Verification items for the finished model (mm, model axes). A direction names the side the tool comes from. Coordinates: 2 decimals unless noted, no trailing zeros. Write each loop counter-clockwise with the first axis right and the second up, starting at its lowest first coordinate (ties: lowest second). Pieces come first, ordered by that corner, then holes. Notation, with made-up numbers: (-5.5, 2.25) -> (8.5, 2.25) arc R18 cw to (8.5, 6.25) -> close; hole circle Ø6 at (16, 32). An arc over 180 degrees is marked (long way). Answer in a Markdown table with one row per item.
Autodesk Inventor part; units mm, degrees
ref_plane "YZ Plane" through (0, 0, 0) normal (1, 0, 0) x (0, 1, 0)
ref_plane "XZ Plane" through (0, 0, 0) normal (0, 1, 0) x (-1, 0, 0)
ref_plane "XY Plane" through (0, 0, 0) normal (0, 0, 1) x (1, 0, 0)
sketch "스케치1" plane through (0, 0, 0) normal (0, 1, 0) x (-1, 0, 0)
  line L0 (0, 0) -> (11.5, 0)
  line L1 (11.5, 0) -> (11.5, -16.1)
  line L2 (11.5, -16.1) -> (0, -16.1)
  line L3 (0, -16.1) -> (0, 0)
  dimension "d0" = 11.5
  dimension "d1" = 16.1
extrude "돌출1" add sketch "스케치1" along normal blind 0.8
fillet "모깎기1" radius 1 2 edges at (0, 0.4, 0) (-11.5, 0.4, 0)
sketch "스케치2" plane through (0, 0.8, 0) normal (0, 1, 0) x (1, 0, 0)
  line L0 (0, 1) -> (0, 16.1)
  line L1 (0, 16.1) -> (-11.5, 16.1)
  line L2 (-1.5, 16.1) -> (-10, 16.1)
  line L3 (-10, 16.1) -> (-10, 14.6)
  line L4 (-10, 14.6) -> (-1.5, 14.6)
  line L5 (-1.5, 14.6) -> (-1.5, 16.1)
  point P0 (0, 0)
  dimension "d5" = 8.5
  dimension "d6" = 1.5
  dimension "d7" = 1.5
extrude "돌출2" add sketch "스케치2" along normal blind 1
properties part number "Case_Top"
1. Sectioned sample at C-C, the plane y = 1.5. Record the cut outline in (x, z), and give its area (4 significant figures).
Findings below:
| item | result |
|---|---|
| outline | (-10, -16.1) -> (-1.5, -16.1) -> (-1.5, -14.6) -> (-10, -14.6) -> close |
| area | 12.75 mm² |
2. Go/stop test with flat-tipped pins: pin 1 (0.5 mm diameter, centred on x = -4.5, y = 1.5, fed in from +Z); pin 2 (0.5 mm diameter, centred on y = 1, z = -15.5, fed in from +X); pin 3 (0.8 mm diameter, centred on y = 1.5, z = -15.5, fed in from -X). Record where each tip stops, or that it passes through.
Findings below:
| item | result |
|---|---|
| pin 1 | stops at z = -14.6 |
| pin 2 | stops at x = 0 |
| pin 3 | stops at x = -10 |
3. Access from +Z, -Z, +X, -X, +Y, -Y to the whole of each face (thin tool, end or side, straight path). Record for faces 1 (the face through (-1.5, 1, -15)), 2 (the face through (-6, 1, -14.6)), 3 (the face through (-10, 1, -15)), 4 (the face through (-6, 1, -16.1)).
Findings below:
| item | result |
|---|---|
| face 1 | +Z, -Z, +X, +Y |
| face 2 | +Z, +X, -X, +Y |
| face 3 | +Z, -Z, -X, +Y |
| face 4 | -Z, +X, -X, +Y, -Y |
4. Sectioned sample at A-A, the plane x = -5.5. Record the cut outline in (y, z).
Findings below:
| item | result |
|---|---|
| outline | (0, -16.1) -> (1.8, -16.1) -> (1.8, -14.6) -> (0.8, -14.6) -> (0.8, 0) -> (0, 0) -> close |
5. Material ranges on probe 1 along Y at (x, z) = (-2.75, -10.25); probe 2 along X at (y, z) = (1, -14.75); probe 3 along Z at (x, y) = (-5.5, 1.5), recorded low to high. Write a range as from..to.
Findings below:
| item | result |
|---|---|
| probe 1 | y = 0..0.8 |
| probe 2 | x = -10..-1.5 |
| probe 3 | z = -16.1..-14.6 |
6. Sectioned sample at B-B, the plane z = -8.25. Record the cut outline in (x, y), and give its area (3 significant figures).
Findings below:
| item | result |
|---|---|
| outline | (-11.5, 0) -> (0, 0) -> (0, 0.8) -> (-11.5, 0.8) -> close |
| area | 9.20 mm² |
